Build history of the part. All positions in model axes, mm. Face numbers are marked on the shaded views. A direction names the side the tool comes from. Round coordinates to 2 decimals unless told otherwise and drop trailing zeros. Loops run counter-clockwise (first coordinate to the right, second up) from the corner with the lowest first, then second, coordinate; pieces in that order, holes last. Notation, with made-up numbers: (36.25, -9.5) - (46.25, -9.5) arc R17 ccw to (46.25, 12.5) - close; hole circle Ø2 at (73, 72.25). An arc over 180 degrees is marked (long way). Use one line per item in the form item = value. Start each with the question number.
Q1. Drill centre lines: line 1 (Z direction, x = 33, y = -17); line 2 (Z direction, x = 32, y = 4); line 3 (X direction, y = 25, z = 0). Where is each one in solid material? Low to high.
Q2. Saw through at B-B (z = 0). Count the separate pieces of the cut face and the enclosed holes in it, then the cut area to 3 significant figures.
Q3. Saw through at A-A (x = 0). Give the cut face in (y, z).
Q4. Pin check, flat tips, straight feed: pin 1 (5 mm diameter, centred on x = 28, y = -1, fed in from -Z); pin 2 (4 mm diameter, centred on y = -7.5, z = 51, fed in from -X); pin 3 (11.5 mm diameter, centred on y = -22.5, z = -0.5, fed in from -X). Stop position of each tip, or through.
Q5. Saw through at C-C (y = -24). Give the cut face in (x, z), then the cut area to 3 significant figures.
Q6. Saw through at D-D (x = 33). Give the cut face in (y, z).
Q7. Mould opens along Z. For the marked faces 4, 5 and 6 say: released by +Z, released by -Z, zero draft, split by the parting line, or undercut.
Q8. 3-axis set-ups, long thin cutter, end or side, ignore diameter. For the marked faces 1, 2 and 3: which of +Z, -Z, +X, -X, +Y, -Y reach the whole face in a straight line?
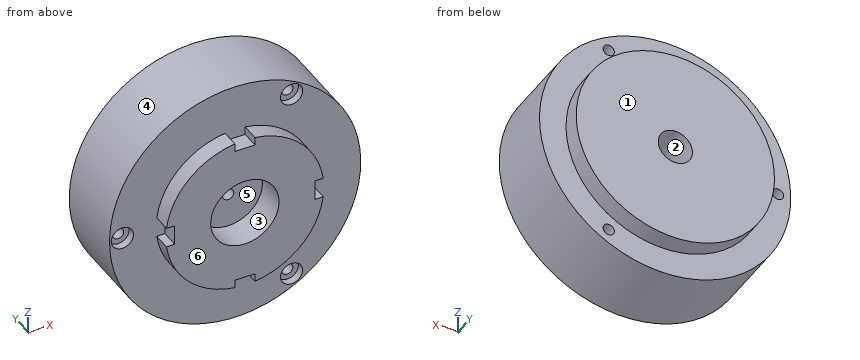
```python
from build123d import *

# Parameters (mm, degrees)
CROQUIS2_R                                           = 10
CORTAR_EXTRUIR1_DEPTH                                = 25
CROQUIS3_R                                           = 20
CORTAR_EXTRUIR2_DEPTH                                = 18
REFRENTADO_PARA_TORNILLO_CON_CABEZA_TRON_D           = 6.6
REFRENTADO_PARA_TORNILLO_CON_CABEZA_TRON_CBORE_D     = 13
REFRENTADO_PARA_TORNILLO_CON_CABEZA_TRON_CBORE_DEPTH = 4.6
CROQUIS6_W                                           = 11.744841144
CROQUIS6_H                                           = 5.153406269
CROQUIS6_W_2                                         = 5.153406269
CROQUIS6_H_2                                         = 11.744841144
CORTAR_EXTRUIR3_DEPTH                                = 10.5


with BuildPart() as part:
    # Croquis1 → Revolución1 (revolve)
    with BuildSketch(Plane.XY, mode=Mode.PRIVATE) as revoluci_n1_sk:
        Polygon((73.5, -19.267048075), (73.5, 24.232951925), (58, 24.232951925), (58, 35.232951925), (0, 35.232951925), (0, -29.767048075), (46.20482663, -29.767048075), (46.20482663, -19.267048075), align=None)
    revolve(revoluci_n1_sk.sketch.rotate(Axis((0, 49.62191358, 0), (0, -1, 0)), 90), axis=Axis((0, 49.62191358, 0), (0, -1, 0)))

    # Croquis2 → Cortar-Extruir1 (cut)
    with BuildSketch(Plane(origin=(0, 35.232951925, 0), x_dir=(1, 0, 0), z_dir=(0, 1, 0))):
        with Locations(Location((0, 0, 0), (0, 0, 270))):
            Circle(CROQUIS2_R)
    extrude(amount=-CORTAR_EXTRUIR1_DEPTH, mode=Mode.SUBTRACT)

    # Croquis3 → Cortar-Extruir2 (cut)
    with BuildSketch(Plane.XZ.offset(29.767048075)):
        with Locations(Location((0, 0, 0), (0, 0, 270))):
            Circle(CROQUIS3_R)
    extrude(amount=-CORTAR_EXTRUIR2_DEPTH, mode=Mode.SUBTRACT)

    # Refrentado para tornillo con cabeza troncocónica de M61 (through all)
    with Locations(Plane(origin=(0, -19.267048075, 0), x_dir=(-1, 0, 0), z_dir=(0, -1, 0))):
        with Locations((66, 0), (-33, -57.15767665), (-33, 57.15767665), (0, 0)):
            CounterBoreHole(REFRENTADO_PARA_TORNILLO_CON_CABEZA_TRON_D / 2, REFRENTADO_PARA_TORNILLO_CON_CABEZA_TRON_CBORE_D / 2, REFRENTADO_PARA_TORNILLO_CON_CABEZA_TRON_CBORE_DEPTH)

    # Croquis6 → Cortar-Extruir3 (cut)
    with BuildSketch(Plane.XZ.offset(29.767048075)):
        with Locations((-0.00913166, -43.646748421)):
            Rectangle(CROQUIS6_W, CROQUIS6_H)
        with Locations((-43.646748421, 0.00913166)):
            Rectangle(CROQUIS6_W_2, CROQUIS6_H_2)
        with Locations((0.00913166, 43.646748421)):
            Rectangle(CROQUIS6_W, CROQUIS6_H)
        with Locations((43.646748421, -0.00913166)):
            Rectangle(CROQUIS6_W_2, CROQUIS6_H_2)
    extrude(amount=-CORTAR_EXTRUIR3_DEPTH, mode=Mode.SUBTRACT)


solid = part.part
```
Report:
q1.line_1 = -65.68 to -63.66, -50.66 to 50.66, 63.66 to 65.68
q1.line_2 = -66.17 to -60.3, -54.01 to 54.01, 60.3 to 66.17
q1.line_3 = -58 to -10, 10 to 58
q2.separate_pieces = 3
q2.enclosed_holes = 0
q2.area = 6,850 mm²
q3.outline = (-29.77, -41.07) - (-19.27, -41.07) - (-19.27, -73.5) - (24.23, -73.5) - (24.23, -58) - (35.23, -58) - (35.23, -10) - (10.23, -10) - (10.23, -3.3) - (-11.77, -3.3) - (-11.77, -20) - (-29.77, -20) - close; (-29.77, 20) - (-11.77, 20) - (-11.77, 3.3) - (10.23, 3.3) - (10.23, 10) - (35.23, 10) - (35.23, 58) - (24.23, 58) - (24.23, 73.5) - (-19.27, 73.5) - (-19.27, 41.07) - (-29.77, 41.07) - close
q4.pin_1 = -68.93
q4.pin_2 = -54.78
q4.pin_3 = -73.5
q5.outline = (-45.83, -5.86) arc R46.2 ccw to (-5.88, -45.83) - (-5.88, -41.07) - (5.86, -41.07) - (5.86, -45.83) arc R46.2 ccw to (45.83, -5.88) - (41.07, -5.88) - (41.07, 5.86) - (45.83, 5.86) arc R46.2 ccw to (5.88, 45.83) - (5.88, 41.07) - (-5.86, 41.07) - (-5.86, 45.83) arc R46.2 ccw to (-45.83, 5.88) - (-41.07, 5.88) - (-41.07, -5.86) - close; hole circle Ø40 at (0, 0)
q5.area = 5,210 mm²
q6.outline = (-29.77, -32.34) - (-19.27, -32.34) - (-19.27, -50.66) - (-14.67, -50.66) - (-14.67, -53.86) - (24.23, -53.86) - (24.23, -47.7) - (35.23, -47.7) - (35.23, 47.7) - (24.23, 47.7) - (24.23, 53.86) - (-14.67, 53.86) - (-14.67, 50.66) - (-19.27, 50.66) - (-19.27, 32.34) - (-29.77, 32.34) - close; (-19.27, -65.68) - (24.23, -65.68) - (24.23, -60.46) - (-14.67, -60.46) - (-14.67, -63.66) - (-19.27, -63.66) - close; (-19.27, 63.66) - (-14.67, 63.66) - (-14.67, 60.46) - (24.23, 60.46) - (24.23, 65.68) - (-19.27, 65.68) - close
q7.face_4 = split by the parting line
q7.face_5 = undercut
q7.face_6 = zero draft
q8.face_1 = +Z, -Z, +X, -X, +Y
q8.face_2 = +Y
q8.face_3 = -Y
